from build123d import *

# Parameters (mm, degrees)
F0_W     = 19.05
F0_H     = 12.7
F1_DEPTH = 19.05


with BuildPart() as f1:
    # F0 (on Front) → F1 (new body)
    with BuildSketch(Plane.XZ):
        Polygon((-152.4, -80.9625), (0, -80.9625), (152.4, -80.9625), (152.4, -71.4375), (133.35, -71.4375), (133.35, -61.9125), (152.4, -61.9125), (152.4, -52.3875), (133.35, -52.3875), (133.35, -42.8625), (152.4, -42.8625), (152.4, -33.3375), (133.35, -33.3375), (133.35, -23.8125), (152.4, -23.8125), (152.4, -14.2875), (133.35, -14.2875), (133.35, -4.7625), (152.4, -4.7625), (152.4, 4.7625), (133.35, 4.7625), (133.35, 14.2875), (152.4, 14.2875), (152.4, 23.8125), (133.35, 23.8125), (133.35, 33.3375), (152.4, 33.3375), (152.4, 42.8625), (133.35, 42.8625), (133.35, 52.3875), (152.4, 52.3875), (152.4, 61.9125), (133.35, 61.9125), (133.35, 71.4375), (152.4, 71.4375), (152.4, 80.9625), (-152.4, 80.9625), (-152.4, 71.4375), (-133.35, 71.4375), (-133.35, 61.9125), (-152.4, 61.9125), (-152.4, 52.3875), (-133.35, 52.3875), (-133.35, 42.8625), (-152.4, 42.8625), (-152.4, 33.3375), (-133.35, 33.3375), (-133.35, 23.8125), (-152.4, 23.8125), (-152.4, 14.2875), (-133.35, 14.2875), (-133.35, 4.7625), (-152.4, 4.7625), (-152.4, -4.7625), (-133.35, -4.7625), (-133.35, -14.2875), (-152.4, -14.2875), (-152.4, -23.8125), (-133.35, -23.8125), (-133.35, -33.3375), (-152.4, -33.3375), (-152.4, -42.8625), (-133.35, -42.8625), (-133.35, -52.3875), (-152.4, -52.3875), (-152.4, -61.9125), (-133.35, -61.9125), (-133.35, -71.4375), (-152.4, -71.4375), align=None)
        with Locations((-89.910227, -25.4)):
            Rectangle(F0_W, F0_H, mode=Mode.SUBTRACT)
        with Locations((86.013636, -25.4)):
            Rectangle(F0_W, F0_H, mode=Mode.SUBTRACT)
        with Locations((-89.910227, 25.4)):
            Rectangle(F0_W, F0_H, mode=Mode.SUBTRACT)
        with Locations((86.013636, 25.4)):
            Rectangle(F0_W, F0_H, mode=Mode.SUBTRACT)
    extrude(amount=F1_DEPTH)


solid = f1.part
The model under review builds one solid part; all positions refer to its coordinate system, in mm. A direction names the side the tool comes from. Coordinates: 2 decimals unless noted, no trailing zeros. Write each loop counter-clockwise with the first axis right and the second up, starting at its lowest first coordinate (ties: lowest second). Pieces come first, ordered by that corner, then holes. Notation, with made-up numbers: (41.5, -15) - (87.5, -15) arc R19 cw to (87.5, 17) - close; hole circle Ø7 at (85.25, -27.75). An arc over 180 degrees is marked (long way). Answer as CSV lines item,"result".
(1) We need section D-D (y = -16). Count the separate pieces of the cut face and the enclosed holes in it, plus the area to 3 significant figures.
Data:
separate pieces,"1"
enclosed holes,"4"
area,"45,500 mm2"
(2) We need section C-C (z = 10). Give the boundary of the cut face in (x, y).
Data:
outline,"(-133.35, -19.05) - (133.35, -19.05) - (133.35, 0) - (-133.35, 0) - close"
(3) We need section B-B (x = -93). Give the boundary of the cut face in (y, z).
Data:
outline,"(-19.05, -80.96) - (0, -80.96) - (0, -31.75) - (-19.05, -31.75) - close; (-19.05, -19.05) - (0, -19.05) - (0, 19.05) - (-19.05, 19.05) - close; (-19.05, 31.75) - (0, 31.75) - (0, 80.96) - (-19.05, 80.96) - close"
(4) For line 1 along Z through (x, y) = (94.5, -12); line 2 along X through (y, z) = (-14.5, -25.5); line 3 along X through (y, z) = (-1.5, 44.5), list the stretches that pass through material, from the lowest coordinate up. Write a range as [from, to].
Data:
line 1,"z = [-80.96, -31.75], [-19.05, 19.05], [31.75, 80.96]"
line 2,"x = [-133.35, -99.44], [-80.39, 76.49], [95.54, 133.35]"
line 3,"x = [-133.35, 133.35]"
(5) Tool access review of faces 1 (the flat face through (143, -9, 61.912)), 2 (the flat face through (-90, -9, -31.75)), 3 (the flat face through (-133.35, -9, -29)), 4 (the flat face through (152.4, -9, -57)): name each direction out of +Z, -Z, +X, -X, +Y, -Y from which nothing blocks a thin tool from reaching the whole face with its end or side.
Data:
face 1,"+X, +Y, -Y"
face 2,"+Y, -Y"
face 3,"-X, +Y, -Y"
face 4,"+Z, -Z, +X, +Y, -Y"
(6) Mouldability with a two-part tool opening along X and no side actions: class faces 5 (the flat face through (152.4, -9, -76)), 6 (the flat face through (-152.4, -9, -76)), 7 (the flat face through (-143, -9, 52.388)), 8 (the flat face through (-99.435, -9, -25)) as pulls with the +X half, pulls with the -X half, needs draft (parallel to the pull), parting line crosses it, or undercut.
Data:
face 5,"pulls with the +X half"
face 6,"pulls with the -X half"
face 7,"needs draft"
face 8,"undercut"
(7) We need section A-A (z = -28). Give the boundary of the cut face in (x, y).
Data:
outline,"(-133.35, -19.05) - (-99.44, -19.05) - (-99.44, 0) - (-133.35, 0) - close; (-80.39, -19.05) - (76.49, -19.05) - (76.49, 0) - (-80.39, 0) - close; (95.54, -19.05) - (133.35, -19.05) - (133.35, 0) - (95.54, 0) - close"
(8) Clearance check with flat-ended pins moving along their axes: pin 1 Ø1 at (y, z) = (-16.5, 25) entering from -X; pin 2 Ø4 at (y, z) = (-12.5, 26) entering from +X. State where each tip first meets the part, or that it passes through.
Data:
pin 1,"stops at x = -133.35"
pin 2,"stops at x = 133.35"
